```python
from build123d import *

# Parameters (mm, degrees)
IZIM1_W                     = 20
IZIM1_H                     = 40
Y_KSEKLIK_EKSTR_ZYON1_DEPTH = 7.5
RADYUS1_R                   = 5
M5_DI_LI_DELIK1_D           = 4.2
M8_DI_LI_DELIK1_D           = 6.8


with BuildPart() as part:
    # Çizim1 → Yükseklik-Ekstrüzyon1 (new, symmetric)
    with BuildSketch(Plane.XY):
        Rectangle(IZIM1_W, IZIM1_H)
    extrude(amount=Y_KSEKLIK_EKSTR_ZYON1_DEPTH, both=True)

    # Radyus1
    radyus1_edges = [part.edges().sort_by_distance(p)[0] for p in [
        (10, -20, 0),
        (-10, -20, 0),
        (-10, 20, 0),
        (10, 20, 0),
    ]]
    fillet(radyus1_edges, radius=RADYUS1_R)

    # M5 Dişli Delik1 (through all)
    with Locations(Plane(origin=(0, 12.5, -7.5), x_dir=(-1, 0, 0), z_dir=(0, 0, -1))):
        with Locations((0, 0), (0, -25)):
            Hole(M5_DI_LI_DELIK1_D / 2)

    # M8 Dişli Delik1 (through all)
    with Locations(Plane.ZY.offset(10)):
        with Locations((0, 0)):
            Hole(M8_DI_LI_DELIK1_D / 2)


solid = part.part
```
For this review, take the finished solid that the model builds, in its own axes (mm). Round coordinates to 2 decimals unless told otherwise and drop trailing zeros. Loops run counter-clockwise (first coordinate to the right, second up) from the corner with the lowest first, then second, coordinate; pieces in that order, holes last.
(1) Wall thickness on line 1 along Y through (x, z) = (0, -3.75); line 2 along Y through (x, z) = (0, 0.25); line 3 along Y through (x, z) = (-1.25, 6.5): over which ranges is each line inside the solid? List them lowest first.
Returned:
line 1: y = -20 to -14.6, -10.4 to 10.4, 14.6 to 20
line 2: y = -20 to -14.6, -10.4 to -3.39, 3.39 to 10.4, 14.6 to 20
line 3: y = -20 to -14.19, -10.81 to 10.81, 14.19 to 20
(2) Mouldability with a two-part tool opening along Z and no side actions: class faces 1 (the cylindrical face through (0.14, -3.32, 0.74)), 2 (the flat face through (0, -20, 0)), 3 (the flat face through (0, 0, 7.5)), 4 (the flat face through (0, 0, -7.5)) as released by +Z, released by -Z, zero draft, split by the parting line, or undercut.
Returned:
face 1: undercut
face 2: zero draft
face 3: released by +Z
face 4: released by -Z
(3) We need section C-C (y = -12.5). Give the boundary of the cut face in (x, z).
Returned:
outline: (-10, -7.5) - (-2.1, -7.5) - (-2.1, 7.5) - (-10, 7.5) - close; (2.1, -7.5) - (10, -7.5) - (10, 7.5) - (2.1, 7.5) - close
(4) We need section B-B (x = 0). Give the boundary of the cut face in (y, z).
Returned:
outline: (-20, -7.5) - (-14.6, -7.5) - (-14.6, 7.5) - (-20, 7.5) - close; (-10.4, -7.5) - (10.4, -7.5) - (10.4, 7.5) - (-10.4, 7.5) - close; (14.6, -7.5) - (20, -7.5) - (20, 7.5) - (14.6, 7.5) - close; hole circle Ø6.8 at (0, 0)
(5) We need section A-A (z = 0). Give the boundary of the cut face in (x, y).
Returned:
outline: (-10, -15) arc R5 ccw to (-5, -20) - (5, -20) arc R5 ccw to (10, -15) - (10, -3.4) - (-10, -3.4) - close; (-10, 3.4) - (10, 3.4) - (10, 15) arc R5 ccw to (5, 20) - (-5, 20) arc R5 ccw to (-10, 15) - close; hole circle Ø4.2 at (0, -12.5); hole circle Ø4.2 at (0, 12.5)
(6) We need section D-D (z = -2.75). Give the boundary of the cut face in (x, y), plus the area to 3 significant figures.
Returned:
outline: (-10, -15) arc R5 ccw to (-5, -20) - (5, -20) arc R5 ccw to (10, -15) - (10, -2) - (-10, -2) - close; (-10, 2) - (10, 2) - (10, 15) arc R5 ccw to (5, 20) - (-5, 20) arc R5 ccw to (-10, 15) - close; hole circle Ø4.2 at (0, -12.5); hole circle Ø4.2 at (0, 12.5)
area: 671 mm2
